Work out the finished part from the listing and answer in its coordinate system (mm). Face numbers are marked on the shaded views. A direction names the side the tool comes from. Coordinates: 2 decimals unless noted, no trailing zeros. Loops run counter-clockwise (first coordinate to the right, second up) from the corner with the lowest first, then second, coordinate; pieces in that order, holes last. Notation, with made-up numbers: (20, 64.5) -> (35, 64.5) arc R18 ccw to (35, 80.5) -> close; hole circle Ø3 at (51, 56.5). An arc over 180 degrees is marked (long way). One line per question, with ' | ' between items.
```python
from build123d import *

# Parameters (mm, degrees)
FILLET1_R       = 0.25
FILLET2_R       = 0.6
HEX_2_DEPTH     = 3
THDSCHPAT_COUNT = 22
THDSCHPAT_PITCH = 1


with BuildPart() as part:
    # BodySke → Base-Revolve (revolve)
    with BuildSketch(Plane.XY):
        Polygon((0, 0), (0, 5), (6, 5), (6, 3), (30.4455, 3), (31, 2.4455), (31, 0), align=None)
    revolve(axis=Axis((-31.75, 0, 0), (1, 0, 0)))

    # Fillet1
    fillet1_edges = [part.edges().sort_by_distance(p)[0] for p in [
        (6, -3, 0),
    ]]
    fillet(fillet1_edges, radius=FILLET1_R)

    # Fillet2
    fillet2_edges = [part.edges().sort_by_distance(p)[0] for p in [
        (0, -5, 0),
    ]]
    fillet(fillet2_edges, radius=FILLET2_R)

    # Sketch2 → Hex-PreBroach (revolve, cut)
    with BuildSketch(Plane.XY):
        Polygon((0, 2.51), (3, 2.51), (4.449149176, 0), (0, 0), align=None)
    revolve(axis=Axis((0, 0, 0), (1, 0, 0)), mode=Mode.SUBTRACT)

    # Sketch3 → Hex 2 (cut)
    with BuildSketch(Plane(origin=(0, 0, 0), x_dir=(0, 0.5, 0.866025404), z_dir=(-1, 0, 0))):
        Polygon((1.449149176, 2.51), (-1.449149176, 2.51), (-2.898298351, 0), (-1.449149176, -2.51), (1.449149176, -2.51), (2.898298351, 0), align=None)
    extrude(amount=-HEX_2_DEPTH, mode=Mode.SUBTRACT)

    # ThdSchSke → ThreadSchematic (revolve, cut)
    with BuildSketch(Plane.XY):
        Polygon((9, -2.4455), (8.61173492, -3), (8.61173492, -3.75), (9.38826508, -3.75), (9.38826508, -3), align=None)
    threadschematic = revolve(axis=Axis((-3.175, 0, 0), (1, 0, 0)), mode=Mode.SUBTRACT)

    # ThdSchPat: ThreadSchematic ×22
    with Locations(*[(i * THDSCHPAT_PITCH, 0, 0) for i in range(1, THDSCHPAT_COUNT)]):
        add(threadschematic, mode=Mode.SUBTRACT)


solid = part.part
```
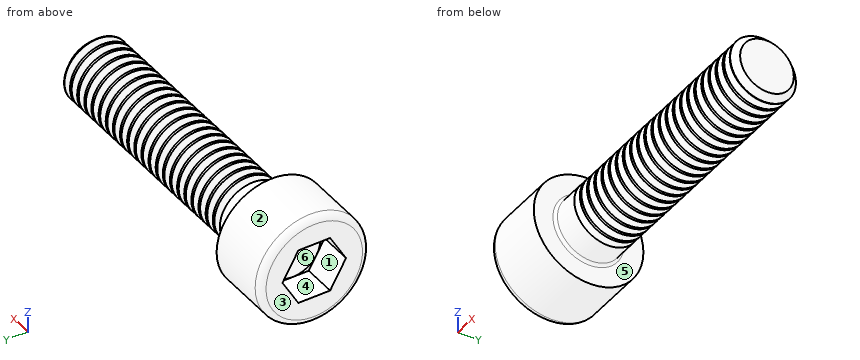
1) Find section A-A (x = 5). Write down the section's boundary in (y, z).
Check values:
outline: circle Ø10 at (0, 0)
2) Find the intervals of material crossed by line 1 along X through (y, z) = (1.5, 3.5); line 2 along Z through (x, y) = (23.5, -0.75); line 3 along Y through (x, z) = (1, 4), in increasing order.
Check values:
line 1: x = 0 to 6 | line 2: z = -2.9 to 2.9 | line 3: y = -3 to 3
3) The mould has two halves that part along Y. Classify the marked faces 1, 2, 3 and 4: released by +Y, released by -Y, zero draft, split by the parting line, or undercut.
Check values:
face 1: undercut | face 2: split by the parting line | face 3: zero draft | face 4: undercut
4) Flat-ended cylindrical pins translate along their axes: pin 1 (1.5 mm diameter, centred on x = 4.5, z = 2.5, fed in from -Y); pin 2 (5 mm diameter, centred on x = 22, y = -4, fed in from -Z); pin 3 (3 mm diameter, centred on x = 27.5, y = -0.5, fed in from +Z). Find the tip coordinate at first contact, or state that the pin passes through.
Check values:
pin 1: stops at y = -4.68 | pin 2: stops at z = -2.58 | pin 3: stops at z = 3
5) For the marked faces 5 and 6, determine the directions among +Z, -Z, +X, -X, +Y, -Y from which every point of the face is accessible in a straight line to the end or side of a thin tool.
Check values:
face 5: +X | face 6: -X
